```python
from build123d import *

# Parameters (mm, degrees)
BOSS_EXTRUDE1_DEPTH         = 4
M4_TAPPED_HOLE1_D           = 3.3
M4_TAPPED_HOLE1_CSINK_D     = 4.85
M4_TAPPED_HOLE1_CSINK_ANGLE = 90
CIRPATTERN1_COUNT           = 8


with BuildPart() as part:
    # Sketch1 → Boss-Extrude1 (new body)
    with BuildSketch(Plane(origin=(0, 0, 0), x_dir=(1, 0, 0), z_dir=(0, 1, 0))):
        with BuildLine():
            Line((0, 33), (0, 42.8))
            ThreePointArc((0, 42.8), (-30.264170235, 30.264170235), (-42.8, 0))
            Line((-42.8, 0), (-33, 0))
            ThreePointArc((-33, 0), (-23.334523779, 23.334523779), (0, 33))
        make_face()
    extrude(amount=BOSS_EXTRUDE1_DEPTH)

    # M4 Tapped Hole1 (through all)
    with Locations(Plane(origin=(0, 4, 0), x_dir=(1, 0, 0), z_dir=(0, 1, 0))):
        with Locations((-35.107422235, 14.54197043)):
            m4_tapped_hole1 = CounterSinkHole(M4_TAPPED_HOLE1_D / 2, M4_TAPPED_HOLE1_CSINK_D / 2, counter_sink_angle=M4_TAPPED_HOLE1_CSINK_ANGLE)

    # CirPattern1: M4 Tapped Hole1 ×8 about axis, 6 skipped
    cirpattern1_axis = Axis((0, 4, 0), (0, 1, 0))
    add([m4_tapped_hole1.rotate(cirpattern1_axis, i * 360 / CIRPATTERN1_COUNT) for i in range(1, CIRPATTERN1_COUNT) if i not in (1, 2, 3, 4, 5, 6)], mode=Mode.SUBTRACT)


solid = part.part
```
Input: part model. Units: mm. Frame: model coordinates. Give positions to 0.01 mm unless a question says otherwise; leave off trailing zeros. Loops run counter-clockwise (first coordinate to the right, second up) from the corner with the lowest first, then second, coordinate; pieces in that order, holes last. Notation, with made-up numbers: (23, -15) -> (72, -15) arc R24 ccw to (72, 20) -> close; hole circle Ø4 at (64, -23.75). An arc over 180 degrees is marked (long way). Use a Markdown table: item, result.
Q1. Ray query, probe 1 along Z at (x, y) = (-36.5, 0.45); probe 2 along Z at (x, y) = (-35, 3.8); probe 3 along X at (y, z) = (2.7, -30). Return the intervals inside material, ascending. Write a range as from..to.
Entries:
| item | result |
|---|---|
| probe 1 | z = -22.35..-15.43, -13.66..0 |
| probe 2 | z = -24.63..-16.76, -12.32..0 |
| probe 3 | x = -30.53..-13.75 |
Q2. Pull-direction query (X, two-part tool) for faces 1 (the flat face through (-25, 0, -25)), 2 (the cylindrical face through (-29.93, 1.972, -30.595)), 3 (the cylindrical face through (-15.4, 1.6, -33.7)); classes: pulls with the +X half, pulls with the -X half, needs draft (parallel to the pull), parting line crosses it, or undercut.
Entries:
| item | result |
|---|---|
| face 1 | needs draft |
| face 2 | pulls with the -X half |
| face 3 | undercut |
Q3. First-contact query: P1, Ø1, axis at x = -8.5, y = 0.5, coming from the +Z side; P2, Ø1.5, axis at x = -14.5, y = 1, coming from the -Z side. Flat tips, straight axial feed; report the tip coordinate or a pass-through.
Entries:
| item | result |
|---|---|
| P1 | stops at z = -31.75 |
| P2 | stops at z = -40.53 |
Q4. Section query A-A, the plane y = 2.55. Return the cut outline in (x, z), plus the area to 3 significant figures.
Entries:
| item | result |
|---|---|
| outline | (-42.8, 0) arc R42.8 ccw to (0, -42.8) -> (0, -33) arc R33 cw to (-33, 0) -> close; hole circle Ø3.3 at (-35.11, -14.54); hole circle Ø3.3 at (-14.54, -35.11) |
| area | 566 mm² |
Q5. Section query C-C, the plane z = -25. Return the cut outline in (x, y), plus the area to 3 significant figures.
Entries:
| item | result |
|---|---|
| outline | (-34.74, 0) -> (-21.54, 0) -> (-21.54, 4) -> (-34.74, 4) -> close |
| area | 52.8 mm² |
Q6. Section query B-B, the plane x = -32. Return the cut outline in (y, z).
Entries:
| item | result |
|---|---|
| outline | (0, -28.42) -> (4, -28.42) -> (4, -8.06) -> (0, -8.06) -> close |
